Work out the finished part from the listing and answer in its coordinate system (mm). A direction names the side the tool comes from. Give positions to 0.01 mm unless a question says otherwise; leave off trailing zeros. Order: outer loops, then holes, each group sorted by start corner. A loop starts at its lowest first (then second) coordinate and runs counter-clockwise, first axis right, second up. Notation, with made-up numbers: (54, 81.5) -> (76, 81.5) arc R30 cw to (76, 111.5) -> close; hole circle Ø9 at (38, 48). An arc over 180 degrees is marked (long way). Answer as CSV lines item,"result". Start each with the question number.
1. A cutting plane is placed at B-B (z = 0.6). Give the vertices of the cut face in (x, y), then the cut area to 3 significant figures.
2. A cutting plane is placed at C-C (y = -4). Give the vertices of the cut face in (x, z), then the cut area to 3 significant figures.
3. A cutting plane is placed at A-A (x = -13). Give the vertices of the cut face in (y, z), then the cut area to 3 significant figures.
4. A cutting plane is placed at D-D (y = 0). Give the vertices of the cut face in (x, z), then the cut area to 3 significant figures.
5. For a pull along Y with two mould halves and no side action, classify faces 1 (the flat face through (0, 0, 0)), 2 (the cylindrical face through (-8.23, 1.5, 0.41)) as released by +Y, released by -Y, zero draft, split by the parting line, or undercut.
6. A flat-ended cylindrical pin translates along its axis: pin 1 (2 mm diameter, centred on x = 0, y = 4, fed in from +Z). Find the tip coordinate at first contact, or state that the pin passes through.
7. Find the intervals of material crossed by L1, parallel to Y at x = -13, z = 0.3; L2, parallel to Y at x = -11, z = 0.4; L3, parallel to X at y = 1.5, z = 0.3, in increasing order.
8. For faces 3 (the flat face through (13, 0, 0.8)), 4 (the flat face through (0, 0, 0.4)), determine the directions among +Z, -Z, +X, -X, +Y, -Y from which every point of the face is accessible in a straight line to the end or side of a thin tool.
from build123d import *

# Parameters (mm, degrees)
F0_W     = 50
F0_H     = 20
F1_DEPTH = 0.4
F2_W     = 23
F2_H     = 20
F3_DEPTH = 0.4
F4_R     = 5
F5_DEPTH = 25


with BuildPart() as f1:
    # F0 (on Top) → F1 (new body)
    with BuildSketch(Plane.XY):
        Rectangle(F0_W, F0_H)
    extrude(amount=F1_DEPTH)

    # F2 (on face) → F3 (join)
    with BuildSketch(Plane.XY.offset(0.4)):
        with Locations((-13.5, 0)):
            Rectangle(F2_W, F2_H)
        with Locations((13.5, 0)):
            Rectangle(F2_W, F2_H)
    extrude(amount=F3_DEPTH)

    # F4 (on face) → F5 (cut)
    with BuildSketch(Plane.XY.offset(0.8)):
        with Locations((-13, 0)):
            Circle(F4_R)
    extrude(amount=-F5_DEPTH, mode=Mode.SUBTRACT)


solid = f1.part
Answer sheet:
1,outline,"(-25, -10) -> (-2, -10) -> (-2, 10) -> (-25, 10) -> close; (2, -10) -> (25, -10) -> (25, 10) -> (2, 10) -> close; hole circle Ø10 at (-13, 0)"
1,area,"841 mm^2"
2,outline,"(-25, 0) -> (-16, 0) -> (-16, 0.8) -> (-25, 0.8) -> close; (-10, 0) -> (25, 0) -> (25, 0.8) -> (2, 0.8) -> (2, 0.4) -> (-2, 0.4) -> (-2, 0.8) -> (-10, 0.8) -> close"
2,area,"33.6 mm^2"
3,outline,"(-10, 0) -> (-5, 0) -> (-5, 0.8) -> (-10, 0.8) -> close; (5, 0) -> (10, 0) -> (10, 0.8) -> (5, 0.8) -> close"
3,area,"8.00 mm^2"
4,outline,"(-25, 0) -> (-18, 0) -> (-18, 0.8) -> (-25, 0.8) -> close; (-8, 0) -> (25, 0) -> (25, 0.8) -> (2, 0.8) -> (2, 0.4) -> (-2, 0.4) -> (-2, 0.8) -> (-8, 0.8) -> close"
4,area,"30.4 mm^2"
5,face 1,"zero draft"
5,face 2,"undercut"
6,pin 1,"stops at z = 0.4"
7,L1,"y = -10 to -5, 5 to 10"
7,L2,"y = -10 to -4.58, 4.58 to 10"
7,L3,"x = -25 to -17.77, -8.23 to 25"
8,face 3,"+Z, +X, -X, +Y, -Y"
8,face 4,"+Z, +Y, -Y"
